Build history of the part. All positions in model axes, mm. Face numbers are marked on the shaded views. A direction names the side the tool comes from. Coordinates: 2 decimals unless noted, no trailing zeros. Loops run counter-clockwise (first coordinate to the right, second up) from the corner with the lowest first, then second, coordinate; pieces in that order, holes last.
Item 1: Drill centre lines: line 1 along Z through (x, y) = (-3.5, -1.25); line 2 along X through (y, z) = (-5, -18); line 3 along Y through (x, z) = (0, 36.6). Where is each one in solid material? Low to high.
Item 2: Flat gauge pins, fed straight in: pin 1 (6 mm diameter, centred on y = -7, z = 28, fed in from +X); pin 2 (1.5 mm diameter, centred on y = -3, z = -30.5, fed in from -X); pin 3 (4 mm diameter, centred on x = 31, y = -4.5, fed in from -Z). Where does each tip first touch, or does it go through?
Item 3: Cut at D-D (x = 18.5). List the corners of the cut face in (y, z).
Item 4: Cut at A-A (x = -19.5). List the corners of the cut face in (y, z).
Item 5: 3-axis set-ups, long thin cutter, end or side, ignore diameter. For the marked faces 1 and 2: which of +Z, -Z, +X, -X, +Y, -Y reach the whole face in a straight line?
Item 6: Cut at B-B (z = 0). Count the separate pieces of the cut face and the enclosed holes in it, and give its area (3 significant figures).
Item 7: Mould opens along X. For the marked faces 3, 4 and 5 say: released by +X, released by -X, zero draft, split by the parting line, or undercut.
from build123d import *

# Parameters (mm, degrees)
SKETCH6_W               = 69
SKETCH6_H               = 69
BOSS_EXTRUDE1_DEPTH     = 10
SKETCH5_R               = 2.25
CUT_EXTRUDE1_DEPTH      = 1
CUT_EXTRUDE1_DEPTH_BACK = 11
CUT_EXTRUDE2_START      = -2
SKETCH7_W               = 56
SKETCH7_H               = 56
CUT_EXTRUDE2_DEPTH      = 10
SKETCH9_W               = 46
SKETCH9_H               = 46
CUT_EXTRUDE3_DEPTH      = 1
CUT_EXTRUDE3_DEPTH_BACK = 11
FILLET1_R               = 10
SKETCH10_R              = 4.5
BOSS_EXTRUDE2_DEPTH     = 4
SKETCH11_R              = 2.5
CUT_EXTRUDE4_DEPTH      = 10.5
SKETCH12_W              = 9.294754328
SKETCH12_H              = 3.5
CUT_EXTRUDE5_DEPTH      = 9
CIRPATTERN1_COUNT       = 4


with BuildPart() as part:
    # Sketch6 → Boss-Extrude1 (new body)
    with BuildSketch(Plane(origin=(0, 0, 0), x_dir=(1, 0, 0), z_dir=(0, 1, 0))):
        Rectangle(SKETCH6_W, SKETCH6_H)
    extrude(amount=-BOSS_EXTRUDE1_DEPTH)

    # Sketch5 → Cut-Extrude1 (cut, two sides)
    with BuildSketch(Plane(origin=(0, 0, 0), x_dir=(1, 0, 0), z_dir=(0, 1, 0))) as cut_extrude1_sk:
        with Locations((27.5, 27.5)):
            Circle(SKETCH5_R)
        with Locations((27.5, -27.5)):
            Circle(SKETCH5_R)
        with Locations((-27.5, -27.5)):
            Circle(SKETCH5_R)
        with Locations((-27.5, 27.5)):
            Circle(SKETCH5_R)
    extrude(amount=CUT_EXTRUDE1_DEPTH, mode=Mode.SUBTRACT)
    extrude(cut_extrude1_sk.sketch, amount=-CUT_EXTRUDE1_DEPTH_BACK, mode=Mode.SUBTRACT)

    # Sketch7 → Cut-Extrude2 (cut)
    with BuildSketch(Plane(origin=(0, 0, 0), x_dir=(1, 0, 0), z_dir=(0, 1, 0)).offset(CUT_EXTRUDE2_START)):
        Rectangle(SKETCH7_W, SKETCH7_H)
    extrude(amount=-CUT_EXTRUDE2_DEPTH, mode=Mode.SUBTRACT)

    # Sketch9 → Cut-Extrude3 (cut, two sides)
    with BuildSketch(Plane(origin=(0, 0, 0), x_dir=(1, 0, 0), z_dir=(0, 1, 0))) as cut_extrude3_sk:
        Rectangle(SKETCH9_W, SKETCH9_H)
    extrude(amount=CUT_EXTRUDE3_DEPTH, mode=Mode.SUBTRACT)
    extrude(cut_extrude3_sk.sketch, amount=-CUT_EXTRUDE3_DEPTH_BACK, mode=Mode.SUBTRACT)

    # Fillet1
    fillet1_edges = [part.edges().sort_by_distance(p)[0] for p in [
        (23, -1, -23),
        (23, -1, 23),
        (-23, -1, 23),
        (-23, -1, -23),
    ]]
    fillet(fillet1_edges, radius=FILLET1_R)

    # Sketch10 → Boss-Extrude2 (add)
    with BuildSketch(Plane(origin=(0, 0, -34.5), x_dir=(-1, 0, 0), z_dir=(0, 0, -1))):
        with Locations((0, -5)):
            Circle(SKETCH10_R)
    boss_extrude2 = extrude(amount=BOSS_EXTRUDE2_DEPTH)

    # Sketch11 → Cut-Extrude4 (cut)
    with BuildSketch(Plane(origin=(0, 0, -38.5), x_dir=(-1, 0, 0), z_dir=(0, 0, -1))):
        with Locations((0, -5)):
            Circle(SKETCH11_R)
    cut_extrude4 = extrude(amount=-CUT_EXTRUDE4_DEPTH, mode=Mode.SUBTRACT)

    # Sketch12 → Cut-Extrude5 (cut)
    with BuildSketch(Plane(origin=(0, -10, 0), x_dir=(-1, 0, 0), z_dir=(0, -1, 0))):
        with Locations((0, 31.188993475)):
            Rectangle(SKETCH12_W, SKETCH12_H)
    cut_extrude5 = extrude(amount=-CUT_EXTRUDE5_DEPTH, mode=Mode.SUBTRACT)

    # CirPattern1: Boss-Extrude2, Cut-Extrude4, Cut-Extrude5 ×4 about axis
    cirpattern1_axis = Axis((0, 0, 0), (0, 1, 0))
    for i in range(1, CIRPATTERN1_COUNT):
        add(boss_extrude2.rotate(cirpattern1_axis, i * 360 / CIRPATTERN1_COUNT))
        add(cut_extrude4.rotate(cirpattern1_axis, i * 360 / CIRPATTERN1_COUNT), mode=Mode.SUBTRACT)
        add(cut_extrude5.rotate(cirpattern1_axis, i * 360 / CIRPATTERN1_COUNT), mode=Mode.SUBTRACT)


solid = part.part
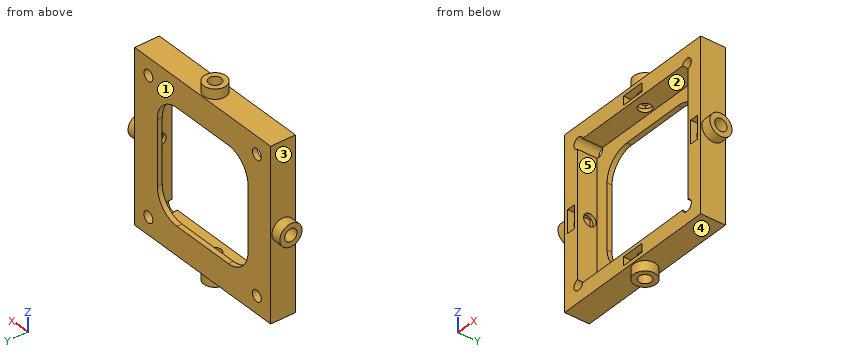
Filled sheet:
1. line 1: z = -34.5 to -32.94, -29.44 to -23, 23 to 29.44, 32.94 to 34.5
1. line 2: x = -34.5 to -28, 28 to 34.5
1. line 3: y = -9.5 to -7.5, -2.5 to -0.5
2. pin 1: stops at x = 34.5
2. pin 2: stops at x = -34.5
2. pin 3: stops at z = -34.5
3. outline: (-10, -34.5) - (0, -34.5) - (0, -21.35) - (-2, -21.35) - (-2, -28) - (-10, -28) - close; (-10, 28) - (-2, 28) - (-2, 21.35) - (0, 21.35) - (0, 34.5) - (-10, 34.5) - close
4. outline: (-10, -34.5) - (0, -34.5) - (0, -20.6) - (-2, -20.6) - (-2, -28) - (-10, -28) - close; (-10, 28) - (-2, 28) - (-2, 20.6) - (0, 20.6) - (0, 34.5) - (-10, 34.5) - close
5. face 1: +Z, -Z, +X, -X, +Y
5. face 2: -Y
6. separate pieces: 6
6. enclosed holes: 0
6. area: 89.0 mm2
7. face 3: released by -X
7. face 4: zero draft
7. face 5: undercut
